```python
from build123d import *

# Parameters (mm, degrees)
F2_R     = 1.25
F3_DEPTH = 12.6


with BuildPart() as f1:
    # F0 (on Front) → F1 (revolve)
    with BuildSketch(Plane.XZ):
        Polygon((-2, 15), (-3.5, 17), (-4.25, 17), (-4.25, 20), (-6.55, 20), (-6.55, 0), (-3, 0), (-3, 2), (-2, 2), align=None)
    revolve(axis=Axis((0, 0, 17.224411), (0, 0, 1)))

    # F2 (on Front) → F3 (cut)
    with BuildSketch(Plane.XZ):
        with Locations((0, 7.5)):
            Circle(F2_R)
    extrude(amount=F3_DEPTH, mode=Mode.SUBTRACT)


solid = f1.part
```
CAD build for the part. Positions are in the model's coordinates, mm. A direction names the side the tool comes from. Give positions to 0.01 mm unless a question says otherwise; leave off trailing zeros. Order: outer loops, then holes, each group sorted by start corner. A loop starts at its lowest first (then second) coordinate and runs counter-clockwise, first axis right, second up.
(1) Flat gauge pins, fed straight in: pin 1 (5.5 mm diameter, centred on x = 0, y = 0, fed in from +Z); pin 2 (1.5 mm diameter, centred on y = 3.5, z = 10.5, fed in from -X); pin 3 (1.5 mm diameter, centred on y = -2, z = 6, fed in from +X). Where does each tip first touch, or does it go through?
(2) Saw through at B-B, the plane y = 0. Give the cut face in (x, z).
(3) Saw through at D-D, the plane z = 7.5. Give the cut face in (x, y).
(4) Saw through at A-A, the plane x = 0. Give the cut face in (y, z).
(5) Mould opens along Y. For faces 3 (the cylindrical face through (-2.285, -3.584, 18.521)), 4 (the cylindrical face through (1.4, 6.4, 9.9)), 5 (the cylindrical face through (-1.25, -4.02, 7.55)) say: released by +Y, released by -Y, zero draft, split by the parting line, or undercut.
(6) Saw through at C-C, the plane y = -4.5. Give the cut face in (x, z).
(7) Tool access for faces 1 (the cylindrical face through (3, 0, 1)), 2 (the flat face through (-3, 1, 0)): list every direction of +Z, -Z, +X, -X, +Y, -Y with a clear straight run to the whole face (end or side of a thin tool).
(8) Drill centre lines: L1, parallel to X at y = 0, z = 9.75; L2, parallel to Z at x = 0, y = -5.5. Where is each one in solid material? Low to high.
Results found:
1. pin 1: stops at z = 16
1. pin 2: stops at x = -5.94
1. pin 3: stops at x = 6.43
2. outline: (-6.55, 0) - (-3, 0) - (-3, 2) - (-2, 2) - (-2, 15) - (-3.5, 17) - (-4.25, 17) - (-4.25, 20) - (-6.55, 20) - close; (2, 2) - (3, 2) - (3, 0) - (6.55, 0) - (6.55, 20) - (4.25, 20) - (4.25, 17) - (3.5, 17) - (2, 15) - close
3. outline: (-1.25, -6.43) - (-1.25, -1.56) arc R2 cw (long way) to (1.25, -1.56) - (1.25, -6.43) arc R6.55 ccw (long way) to start
4. outline: (-6.55, 0) - (-3, 0) - (-3, 2) - (-2, 2) - (-2, 6.25) - (-6.55, 6.25) - close; (-6.55, 8.75) - (-2, 8.75) - (-2, 15) - (-3.5, 17) - (-4.25, 17) - (-4.25, 20) - (-6.55, 20) - close; (2, 2) - (3, 2) - (3, 0) - (6.55, 0) - (6.55, 20) - (4.25, 20) - (4.25, 17) - (3.5, 17) - (2, 15) - close
5. face 3: undercut
5. face 4: split by the parting line
5. face 5: zero draft
6. outline: (-4.76, 0) - (4.76, 0) - (4.76, 20) - (-4.76, 20) - close; hole circle Ø2.5 at (0, 7.5)
7. face 1: -Z
7. face 2: -Z, +X, -X, +Y, -Y
8. L1: x = -6.55 to -2, 2 to 6.55
8. L2: z = 0 to 6.25, 8.75 to 20
